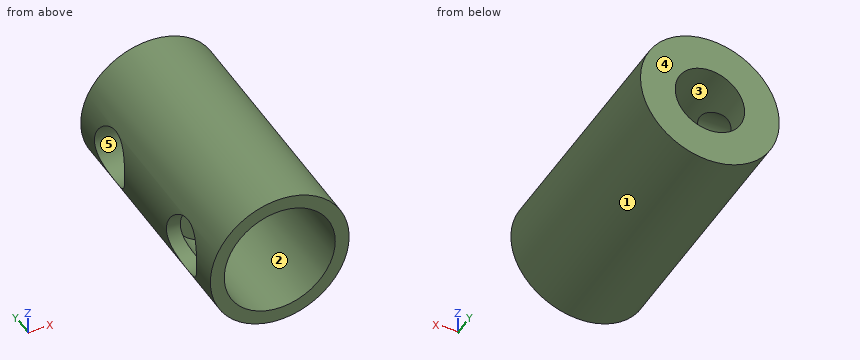
from build123d import *

# Parameters (mm, degrees)
F0_R     = 5
F1_DEPTH = 18
F2_R     = 4
F3_DEPTH = 8
F4_R     = 2.5
F5_DEPTH = 8
F7_D     = 4.2
F7_DEPTH = 14.4
F7_TIP   = 1.2618073
F8_D     = 4.2
F8_DEPTH = 14.4
F8_TIP   = 1.2618073


with BuildPart() as f1:
    # F0 (on Front) → F1 (new body)
    with BuildSketch(Plane.XZ):
        Circle(F0_R)
    extrude(amount=F1_DEPTH)

    # F2 (on face) → F3 (cut)
    with BuildSketch(Plane.XZ.offset(18)):
        Circle(F2_R)
    extrude(amount=-F3_DEPTH, mode=Mode.SUBTRACT)

    # F4 (on face) → F5 (cut)
    with BuildSketch(Plane(origin=(0, 0, 0), x_dir=(-1, 0, 0), z_dir=(0, 1, 0))):
        Circle(F4_R)
    extrude(amount=-F5_DEPTH, mode=Mode.SUBTRACT)

    # F7 (one way)
    with BuildSketch(Plane.YZ):
        with Locations((-4, 0)):
            Circle(F7_D / 2)
    extrude(amount=-F7_DEPTH, mode=Mode.SUBTRACT)
    with Locations(Plane.YZ):
        with Locations((-4, 0)):
            with Locations((0, 0, -(F7_DEPTH + F7_TIP / 2))):  # 118° drill point
                Cone(0, F7_D / 2, F7_TIP, mode=Mode.SUBTRACT)

    # F8 (one way)
    with BuildSketch(Plane.YZ):
        with Locations((-14, 0)):
            Circle(F8_D / 2)
    extrude(amount=-F8_DEPTH, mode=Mode.SUBTRACT)
    with Locations(Plane.YZ):
        with Locations((-14, 0)):
            with Locations((0, 0, -(F8_DEPTH + F8_TIP / 2))):  # 118° drill point
                Cone(0, F8_D / 2, F8_TIP, mode=Mode.SUBTRACT)


solid = f1.part
Input: part model. Units: mm. Frame: model coordinates. Face numbers are marked on the shaded views. A direction names the side the tool comes from. Coordinates: 2 decimals unless noted, no trailing zeros. Loops run counter-clockwise (first coordinate to the right, second up) from the corner with the lowest first, then second, coordinate; pieces in that order, holes last.
(1) Section C-C on y = -7.75. Return the cut outline in (x, z).
(2) Section B-B on x = 0. Return the cut outline in (y, z), then the cut area to 3 significant figures.
(3) Material intervals for probe 1 along Z at (x, y) = (0, -5.5); probe 2 along Y at (x, z) = (1, 1.5); probe 3 along Y at (x, z) = (1.75, -3.25), sorted ascending.
(4) Section A-A on z = 0. Return the cut outline in (x, y), then the cut area to 3 significant figures.
(5) Set-up query: the marked faces 1, 2 and 3. Return all of +Z, -Z, +X, -X, +Y, -Y with unobstructed straight access to the full face (end or side cutting, diameter ignored); none if empty.
(6) Pull-direction query (Y, two-part tool) for the marked faces 4 and 5; classes: released by +Y, released by -Y, zero draft, split by the parting line, or undercut.
(7) First-contact query: pin 1 Ø6 at (x, z) = (0, -2.5) entering from +Y; pin 2 Ø1.5 at (x, z) = (0, 0) entering from +Y; pin 3 Ø4 at (x, z) = (0, 0) entering from -Y; pin 4 Ø6 at (x, y) = (4, -15) entering from -Z. Flat tips, straight axial feed; report the tip coordinate or a pass-through.
(8) Section D-D on z = 3. Return the cut outline in (x, y), then the cut area to 3 significant figures.
Data:
1. outline: circle Ø10 at (0, 0); hole circle Ø5 at (0, 0)
2. outline: (-18, -5) - (0, -5) - (0, -2.5) - (-8, -2.5) - (-8, 2.5) - (0, 2.5) - (0, 5) - (-18, 5) - (-18, 4) - (-10, 4) - (-10, -4) - (-18, -4) - close
2. area: 76.0 mm2
3. probe 1: z = -5 to -2.5, 2.5 to 5
3. probe 2: y = -10 to -8
3. probe 3: y = -10 to 0
4. outline: (-5, -18) - (-4, -18) - (-4, -16.1) - (-5, -16.1) - close; (-5, -11.9) - (-4, -11.9) - (-4, -10) - (4, -10) - (4, -18) - (5, -18) - (5, 0) - (2.5, 0) - (2.5, -8) - (-2.5, -8) - (-2.5, -6.1) - (-5, -6.1) - close; (-5, -1.9) - (-2.5, -1.9) - (-2.5, 0) - (-5, 0) - close
4. area: 61.3 mm2
5. face 1: +Y, -Y
5. face 2: -Y
5. face 3: +Y
6. face 4: released by +Y
6. face 5: undercut
7. pin 1: stops at y = 0
7. pin 2: stops at y = -8
7. pin 3: stops at y = -10
7. pin 4: stops at z = -4.9
8. outline: (-4, -18) - (-2.65, -18) - (-2.65, -10) - (2.65, -10) - (2.65, -18) - (4, -18) - (4, 0) - (-4, 0) - close
8. area: 102 mm2
